```python
from build123d import *

# Parameters (mm, degrees)
F0_R        = 3.5
F1_DEPTH    = 25
F2_T1_DEPTH = 35.23561564
F2_T3_DEPTH = 35.4401476299


# Not quite as in the source:
# - a fillet or chamfer that OpenCascade refuses, or shapes differently, is made with other operations: its cross-section is extruded or revolved along the edge and cut away or added


with BuildPart() as f1:
    # F0 (on Top) → F1 (new body)
    with BuildSketch(Plane.XY):
        with BuildLine():
            ThreePointArc((23.5, 4.5), (20.3180194847, 3.1819805153), (19, 0))
            ThreePointArc((19, 0), (20.3180194847, -3.1819805153), (23.5, -4.5))
            ThreePointArc((23.5, -4.5), (26.6819805153, -3.1819805153), (28, 0))
            ThreePointArc((28, 0), (26.6819805153, 3.1819805153), (23.5, 4.5))
        make_face()
        with Locations((23.5, 0)):
            Circle(F0_R, mode=Mode.SUBTRACT)
        with BuildLine():
            ThreePointArc((18.459414942, 4.5), (18.8643696409, 2.2661769682), (19, 0))
            ThreePointArc((19, 0), (20.3180194847, 3.1819805153), (23.5, 4.5))
            Line((23.5, 4.5), (18.459414942, 4.5))
        make_face()
        with BuildLine():
            ThreePointArc((23.5, -4.5), (20.3180194847, -3.1819805153), (19, 0))
            ThreePointArc((19, 0), (18.8643696409, -2.2661769682), (18.459414942, -4.5))
            Line((18.459414942, -4.5), (23.5, -4.5))
        make_face()
        with BuildLine():
            ThreePointArc((18.459414942, -4.5), (18.8643696409, -2.2661769682), (19, 0))
            ThreePointArc((19, 0), (18.8643696409, 2.2661769682), (18.459414942, 4.5))
            ThreePointArc((18.459414942, 4.5), (18.1842599773, 5.507512059), (17.8541597949, 6.4983827232))
            Line((17.8541597949, 6.4983827232), (16.9144671741, 6.1563625799))
            ThreePointArc((16.9144671741, 6.1563625799), (17.7265395542, 3.125667198), (18, 0))
            ThreePointArc((18, 0), (17.7265395542, -3.125667198), (16.9144671741, -6.1563625799))
            Line((16.9144671741, -6.1563625799), (17.8541597949, -6.4983827232))
            ThreePointArc((17.8541597949, -6.4983827232), (18.1842599773, -5.507512059), (18.459414942, -4.5))
        make_face()
    extrude(amount=F1_DEPTH)

    # F2: fillet of radius 2.25 on 2 edges, made by hand

    # F2_s2 → F2_t1 (cut)
    with BuildSketch(Plane.XY.offset(-5.11780782)):
        with BuildLine():
            ThreePointArc((16.9144671741, -6.1563625799), (17.8963613222, -5.5515835221), (18.4496693096, -4.5397910048))
            Line((18.4496693096, -4.5397910048), (18.4933658948, -4.5505431414))
            ThreePointArc((18.4933658948, -4.5505431414), (18.2213657624, -5.5402034939), (17.8964459629, -6.5137736296))
            Line((17.8964459629, -6.5137736296), (17.8387688885, -6.5406688911))
            ThreePointArc((17.8387688885, -6.5406688911), (17.3689225781, -6.3696588195), (16.9274597166, -6.1994461479))
            Line((16.9274597166, -6.1994461479), (16.9144671741, -6.1563625799))
        make_face()
    extrude(amount=F2_T1_DEPTH, mode=Mode.SUBTRACT)

    # F2_s4 → F2_t3 (cut)
    with BuildSketch(Plane.XY.offset(-5.2200738149)):
        with BuildLine():
            ThreePointArc((18.459414942, 4.5), (17.9105670548, 5.5367651403), (16.9144671741, 6.1563625799))
            Line((16.9144671741, 6.1563625799), (16.9274524792, 6.1994483299))
            ThreePointArc((16.9274524792, 6.1994483299), (17.3689225781, 6.3696588195), (17.8387688885, 6.5406688911))
            Line((17.8387688885, 6.5406688911), (17.8964459629, 6.5137736296))
            ThreePointArc((17.8964459629, 6.5137736296), (18.2273279614, 5.5205561665), (18.5032992024, 4.5099584984))
            Line((18.5032992024, 4.5099584984), (18.459414942, 4.5))
        make_face()
    extrude(amount=F2_T3_DEPTH, mode=Mode.SUBTRACT)


solid = f1.part
```
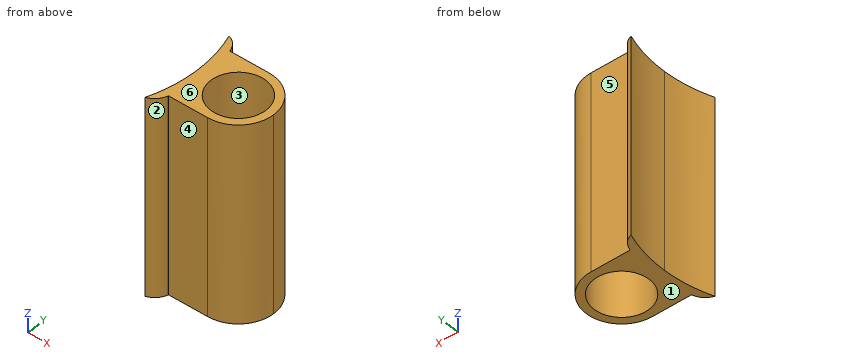
Here's how the part is built. I have some questions about the finished solid (model axes, mm). Face numbers are marked on the shaded views. A direction names the side the tool comes from. Coordinates: 2 decimals unless noted, no trailing zeros. Order: outer loops, then holes, each group sorted by start corner. A loop starts at its lowest first (then second) coordinate and runs counter-clockwise, first axis right, second up.
1) Imagine slicing it at D-D on y = -4. List the corners of the cut face in (x, z) for me.
2) Imagine slicing it at C-C on x = 26.25. List the corners of the cut face in (y, z) for me, and give its area (3 significant figures).
3) Imagine slicing it at B-B on y = 1.75. List the corners of the cut face in (x, z) for me, and give its area (3 significant figures).
4) Which directions (+Z, -Z, +X, -X, +Y, -Y) give clear straight access to the entire face, cutting with the end or side of a thin tool? Please do the marked faces 4, 5 and 6.
5) Imagine slicing it at A-A on z = 21.5. List the corners of the cut face in (x, y) for me, and give its area (3 significant figures).
6) I need wall thicknesses on line 1 (Y direction, x = 23.5, z = 17.5); line 2 (X direction, y = 3, z = 1.75); line 3 (Y direction, x = 25.75, z = 19.5). Which ranges of each line are inside material? Lowest first, please.
7) We'd pull the mould along Y, two halves only. Please class the marked faces 1, 2 and 3: +Y half, -Y half, draft (parallel to the pull), parting line (faces both ways), or undercut.
8) Will these pins go through, and if not, where does the flat tip stop? pin 1 (1.5 mm diameter, centred on x = 21.5, y = -1, fed in from -Z); pin 2 (5 mm diameter, centred on x = 25, z = 12, fed in from +Y); pin 3 (4 mm diameter, centred on x = 21, y = 5, fed in from -Z); pin 4 (1.5 mm diameter, centred on x = 27, z = 14, fed in from -Y).
Response values:
1. outline: (17.55, 0) - (25.56, 0) - (25.56, 25) - (17.55, 25) - close
2. outline: (-3.56, 0) - (-2.17, 0) - (-2.17, 25) - (-3.56, 25) - close; (2.17, 0) - (3.56, 0) - (3.56, 25) - (2.17, 25) - close
2. area: 69.8 mm2
3. outline: (17.91, 0) - (20.47, 0) - (20.47, 25) - (17.91, 25) - close; (26.53, 0) - (27.65, 0) - (27.65, 25) - (26.53, 25) - close
3. area: 91.7 mm2
4. face 4: +Z, -Z, +X, -Y
4. face 5: +Z, -Z, +X, +Y
4. face 6: +Z, +X, -X, +Y, -Y
5. outline: (16.91, -6.16) arc R2.25 ccw to (18.45, -4.54) arc R19 ccw to (18.46, -4.5) - (23.5, -4.5) arc R4.5 ccw to (23.5, 4.5) - (18.46, 4.5) arc R19 ccw to (18.44, 4.58) arc R2.25 ccw to (16.91, 6.16) arc R18 cw to start; hole circle Ø7 at (23.5, 0)
5. area: 47.1 mm2
6. line 1: y = -4.5 to -3.5, 3.5 to 4.5
6. line 2: x = 17.75 to 21.7, 25.3 to 26.85
6. line 3: y = -3.9 to -2.68, 2.68 to 3.9
7. face 1: draft
7. face 2: -Y half
7. face 3: undercut
8. pin 1: passes through
8. pin 2: stops at y = 4.5
8. pin 3: stops at z = 0
8. pin 4: stops at y = -3.56
